Can you work these out from the drawing? Everything is in mm from the part's minimum corner. A direction names the side the tool comes from. Give positions to 0.01 mm unless a question says otherwise; leave off trailing zeros. Write each loop counter-clockwise with the first axis right and the second up, starting at its lowest first coordinate (ties: lowest second). Pieces come first, ordered by that corner, then holes. Notation, with made-up numbers: (-39, -5.75) - (19, -5.75) arc R9 ccw to (19, 10.25) - close; hole circle Ø10 at (71.5, 45.5). An arc over 180 degrees is marked (long way). Use a Markdown table: item, result.
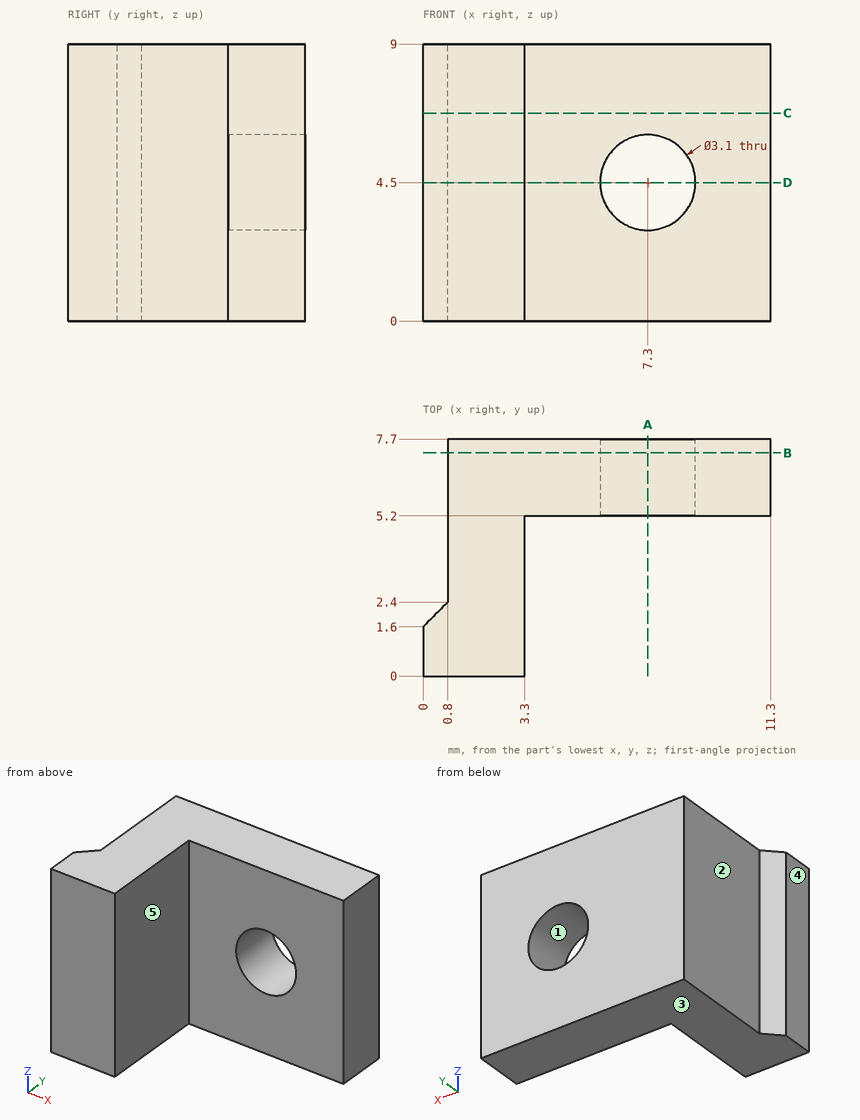
Item 1: If we section it at B-B, the plane y = 7.25: Write out the boundary of the cut face in (x, z).
Values:
| item | result |
|---|---|
| outline | (0.8, 0) - (11.3, 0) - (11.3, 9) - (0.8, 9) - close; hole circle Ø3.1 at (7.3, 4.5) |
Item 2: For the marked faces 4 and 5, which set-ups out of +Z, -Z, +X, -X, +Y, -Y let a thin tool reach every point of the face, with its end or its side?
Values:
| item | result |
|---|---|
| face 4 | +Z, -Z, -X, +Y, -Y |
| face 5 | +Z, -Z, +X, -Y |
Item 3: I need wall thicknesses on line 1 along Z through (x, y) = (7.3, 6.55); line 2 along Y through (x, z) = (3.75, 5); line 3 along X through (y, z) = (3.75, 1). Which ranges of each line are inside material? Lowest first, please. Write a range as [from, to].
Values:
| item | result |
|---|---|
| line 1 | z = [0, 2.95], [6.05, 9] |
| line 2 | y = [5.2, 7.7] |
| line 3 | x = [0.8, 3.3] |
Item 4: If we section it at D-D, the plane z = 4.5: Write out the boundary of the cut face in (x, y), plus the area to 3 significant figures.
Values:
| item | result |
|---|---|
| outline | (0, 0) - (3.3, 0) - (3.3, 5.2) - (5.75, 5.2) - (5.75, 7.7) - (0.8, 7.7) - (0.8, 2.4) - (0, 1.6) - close; (8.85, 5.2) - (11.3, 5.2) - (11.3, 7.7) - (8.85, 7.7) - close |
| area | 33.1 mm2 |
Item 5: Thinking about a two-plate mould opening in Z: for the marked faces 1, 2 and 3, which applies, +Z half, -Z half, draft (parallel to the pull), parting line (faces both ways), or undercut?
Values:
| item | result |
|---|---|
| face 1 | undercut |
| face 2 | draft |
| face 3 | -Z half |
Item 6: If we section it at A-A, the plane x = 7.3: Write out the boundary of the cut face in (y, z), plus the area to 4 significant figures.
Values:
| item | result |
|---|---|
| outline | (5.2, 0) - (7.7, 0) - (7.7, 2.95) - (5.2, 2.95) - close; (5.2, 6.05) - (7.7, 6.05) - (7.7, 9) - (5.2, 9) - close |
| area | 14.75 mm2 |
Item 7: Will these pins go through, and if not, where does the flat tip stop? pin 1 Ø4 at (y, z) = (5, 3.5) entering from +X; pin 2 Ø4 at (y, z) = (5, 3) entering from -X; pin 3 Ø4 at (x, z) = (7.3, 4.5) entering from -Y.
Values:
| item | result |
|---|---|
| pin 1 | stops at x = 11.3 |
| pin 2 | stops at x = 0.8 |
| pin 3 | stops at y = 5.2 |
Item 8: If we section it at C-C, the plane z = 6.75: Write out the boundary of the cut face in (x, y).
Values:
| item | result |
|---|---|
| outline | (0, 0) - (3.3, 0) - (3.3, 5.2) - (11.3, 5.2) - (11.3, 7.7) - (0.8, 7.7) - (0.8, 2.4) - (0, 1.6) - close |
